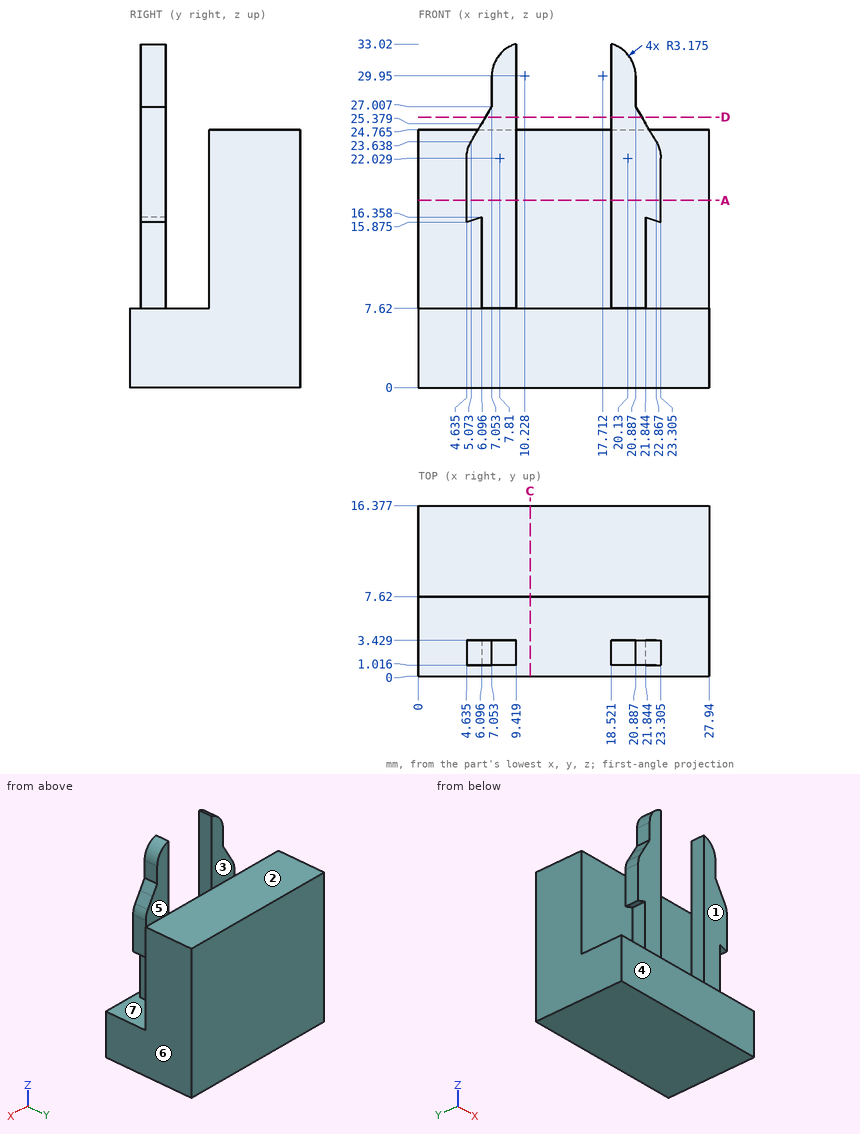
Geometry: see drawing. Coordinates: mm, zero at the bounding-box minimum. A direction names the side the tool comes from. Give positions to 0.01 mm unless a question says otherwise; leave off trailing zeros. Write each loop counter-clockwise with the first axis right and the second up, starting at its lowest first coordinate (ties: lowest second). Pieces come first, ordered by that corner, then holes. Notation, with made-up numbers: M 72,0.25 L 104,0.25 A19 ccw 104,20.25 Z; hole C 53,83 d11. An arc over 180 degrees is marked long. Answer as a JSON object with one key per item and string values.
Q1. Ray query, line 1 along Y through (x, z) = (22.5, 20.5); line 2 along Z through (x, y) = (11, 15.75) (1 decimal); line 3 along Z through (x, y) = (17.25, 1). Return the intervals inside material, ascending.
Geometry check:
{"line 1": "y = 1.02 to 3.43, 7.62 to 16.38", "line 2": "z = 0 to 24.8", "line 3": "z = 0 to 7.62"}
Q2. Contact query for flat-ended pins moving along their axis: P1, Ø1.5, axis at x = 13.5, y = 2.5, coming from the +Z side; P2, Ø8.5, axis at x = 17.5, z = 17, coming from the -Y side; P3, Ø2.5, axis at y = 1.5, z = 18.5, coming from the +X side (1 decimal). Output: stop coordinate, or through.
Geometry check:
{"P1": "stops at z = 7.62", "P2": "stops at y = 1.02", "P3": "stops at x = 23.3"}
Q3. Cut plane D-D, the plane z = 26. Return the cut outline in (x, y), then the cut area to 3 significant figures.
Geometry check:
{"outline": "M 6.46,1.02 L 9.42,1.02 L 9.42,3.43 L 6.46,3.43 Z; M 18.52,1.02 L 21.48,1.02 L 21.48,3.43 L 18.52,3.43 Z", "area": "14.3 mm^2"}
Q4. Mould query, pull axis X, two halves, no side actions, for the marked faces 5, 6 and 7. Classes: +X half, -X half, draft (parallel to the pull), parting line (faces both ways), or undercut.
Geometry check:
{"face 5": "draft", "face 6": "+X half", "face 7": "undercut"}
Q5. Cut plane A-A, the plane z = 18. Return the cut outline in (x, y) (1 decimal).
Geometry check:
{"outline": "M 0,7.6 L 27.9,7.6 L 27.9,16.4 L 0,16.4 Z; M 4.6,1 L 9.4,1 L 9.4,3.4 L 4.6,3.4 Z; M 18.5,1 L 23.3,1 L 23.3,3.4 L 18.5,3.4 Z"}
Q6. Access query for the marked faces 1, 2, 3 and 4. Directions: +Z, -Z, +X, -X, +Y, -Y. A direction counts if a zero-diameter tool reaches every point of the face in a straight line with its end or side. Return the directions, or none.
Geometry check:
{"face 1": "+Z, +X, -X, -Y", "face 2": "+Z, +X, -X, +Y", "face 3": "+Z, +X, -X", "face 4": "+Z, -Z, +X, -X, -Y"}
Q7. Cut plane C-C, the plane x = 10.75. Return the cut outline in (y, z) (1 decimal), then the cut area to 3 significant figures.
Geometry check:
{"outline": "M 0,0 L 16.4,0 L 16.4,24.8 L 7.6,24.8 L 7.6,7.6 L 0,7.6 Z", "area": "275 mm^2"}
